Work out the finished part from the listing and answer in its coordinate system (mm). Give positions to 0.01 mm unless a question says otherwise; leave off trailing zeros. Loops run counter-clockwise (first coordinate to the right, second up) from the corner with the lowest first, then second, coordinate; pieces in that order, holes last. Notation, with made-up numbers: (83.5, 66) - (124.5, 66) arc R13 cw to (124.5, 72) - close; hole circle Ø10 at (76.25, -18). An arc over 180 degrees is marked (long way). One line per question, with ' | ' between items.
from build123d import *

# Parameters (mm, degrees)
SKETCH1_R           = 6.5
SKETCH1_R_2         = 2
BOSS_EXTRUDE1_DEPTH = 5
SKETCH2_R           = 1.6
CUT_EXTRUDE1_DEPTH  = 10


with BuildPart() as part:
    # Sketch1 → Boss-Extrude1 (new body)
    with BuildSketch(Plane.XY):
        with BuildLine():
            Line((0, 12.5), (180, 12.5))
            ThreePointArc((180, 12.5), (192.5, 0), (180, -12.5))
            Line((180, -12.5), (0, -12.5))
            ThreePointArc((0, -12.5), (-12.5, 0), (0, 12.5))
        make_face()
        Circle(SKETCH1_R, mode=Mode.SUBTRACT)
        with Locations((144, 0)):
            Circle(SKETCH1_R_2, mode=Mode.SUBTRACT)
    extrude(amount=BOSS_EXTRUDE1_DEPTH)

    # Sketch2 → Cut-Extrude1 (cut)
    with BuildSketch(Plane.XZ.offset(12.5)):
        with Locations(Location((175, 2.5, 0), (0, 0, 270))):
            Circle(SKETCH2_R)
    extrude(amount=-CUT_EXTRUDE1_DEPTH, mode=Mode.SUBTRACT)


solid = part.part
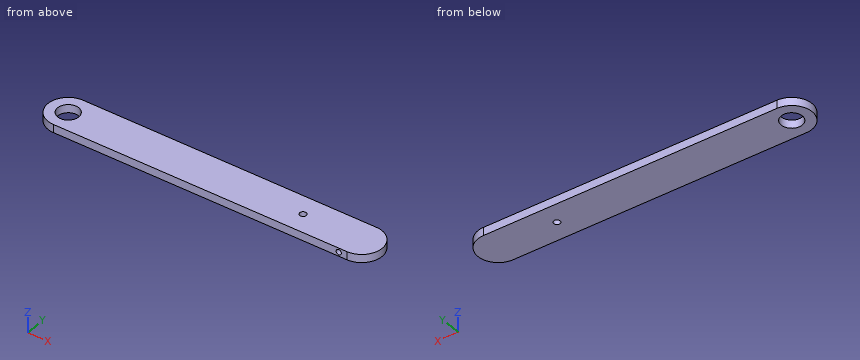
1. Find section A-A on x = 144. Write down the section's boundary in (y, z), then the cut area to 3 significant figures.
Evaluation:
outline: (-12.5, 0) - (-2, 0) - (-2, 5) - (-12.5, 5) - close; (2, 0) - (12.5, 0) - (12.5, 5) - (2, 5) - close | area: 105 mm2
2. Consider L1, parallel to Y at x = 144, z = 1.5; L2, parallel to Z at x = 175, y = -9; L3, parallel to X at y = -0.5, z = 3.95. Determine where each line is inside the solid, lowest interval first.
Evaluation:
L1: -12.5 to -2, 2 to 12.5 | L2: 0 to 0.9, 4.1 to 5 | L3: -12.49 to -6.48, 6.48 to 142.06, 145.94 to 192.49
3. Find section B-B on y = 0. Write down the section's boundary in (x, z), then the cut area to 3 significant figures.
Evaluation:
outline: (-12.5, 0) - (-6.5, 0) - (-6.5, 5) - (-12.5, 5) - close; (6.5, 0) - (142, 0) - (142, 5) - (6.5, 5) - close; (146, 0) - (192.5, 0) - (192.5, 5) - (146, 5) - close | area: 940 mm2
4. Find section D-D on y = -10.5. Write down the section's boundary in (x, z).
Evaluation:
outline: (-6.78, 0) - (186.78, 0) - (186.78, 5) - (-6.78, 5) - close; hole circle Ø3.2 at (175, 2.5)
5. Flat-ended cylindrical pins translate along their axes: pin 1 (2 mm diameter, centred on y = 3.5, z = 4.5, fed in from -X); pin 2 (11.5 mm diameter, centred on x = 0, y = 0, fed in from +Z). Find the tip coordinate at first contact, or state that the pin passes through.
Evaluation:
pin 1: x = -12.25 | pin 2: through
6. Find section C-C on z = 2.5. Write down the section's boundary in (x, y).
Evaluation:
outline: (0, -12.5) - (173.4, -12.5) - (173.4, -2.5) - (176.6, -2.5) - (176.6, -12.5) - (180, -12.5) arc R12.5 ccw to (180, 12.5) - (0, 12.5) arc R12.5 ccw to start; hole circle Ø13 at (0, 0); hole circle Ø4 at (144, 0)
